Verification items for the finished model (mm, model axes). A direction names the side the tool comes from. Give positions to 0.01 mm unless a question says otherwise; leave off trailing zeros. Loops run counter-clockwise (first coordinate to the right, second up) from the corner with the lowest first, then second, coordinate; pieces in that order, holes last. Notation, with made-up numbers: (78, -22.5) - (87, -22.5) arc R24 cw to (87, -5.5) - close; hole circle Ø9 at (60, -35). An arc over 180 degrees is marked (long way). One line per item, written item: value. Start each with the question number.
1. Mould release check, pull along X, two halves, no side actions. Record for faces 1 (the cylindrical face through (19.961, 48.268, 10.382)), 2 (the flat face through (-3.82, 41.5, -22.34)), 3 (the flat face through (-6, 33, 12)): pulls with the +X half, pulls with the -X half, needs draft (parallel to the pull), parting line crosses it, or undercut.
2. Scan lines: L1, parallel to X at y = 17, z = 0; L2, parallel to X at y = 43, z = 0; L3, parallel to Y at x = 11, z = 22. Record each from-to range of solid material in increasing order. Write a range as [from, to].
3. Sectioned sample at C-C (y = 40.5). Record the cut outline in (x, z).
4. Sectioned sample at A-A (y = 30.5). Record the cut outline in (x, z), plus the area to 3 significant figures.
5. Sectioned sample at B-B (z = 14). Count the separate pieces of the cut face and the enclosed holes in it, plus the area to 3 significant figures.
6. Gauge pin test, flat ends, axial feed: pin 1 (10 mm diameter, centred on x = 16, z = 15.5, fed in from +Y); pin 2 (4 mm diameter, centred on x = 16.5, z = -5.5, fed in from -Y); pin 3 (1.5 mm diameter, centred on x = 12.5, y = 16.5, fed in from -Z). Record the tip position at first contact, or that the pin passes through.
7. Access from +Z, -Z, +X, -X, +Y, -Y to the whole of each face (thin tool, end or side, straight path). Record for faces 4 (the flat face through (-6, 33, -12)), 5 (the cylindrical face through (-0.8, 36.7, 18.4)), 6 (the cylindrical face through (-0.319, 23.257, 17.423)).
from build123d import *

# Parameters (mm, degrees)
CUT_EXTRUDE1_DEPTH       = 70
SKETCH3_R                = 6.25
CUT_EXTRUDE2_DEPTH       = 70
BOSS_EXTRUDE2_REACH      = 78.823
BOSS_EXTRUDE2_END_RADIUS = 23
SKETCH4_R                = 7.25
SKETCH4_R_2              = 6.25


with BuildPart() as part:
    # Sketch1 → Revolve1 (revolve)
    with BuildSketch(Plane.XY, mode=Mode.PRIVATE) as revolve1_sk:
        with BuildLine():
            Line((0, 62.5), (0, 60.49936285))
            ThreePointArc((0, 60.49936285), (12.069492637, 58.859165445), (23, 53.484511145))
            Line((23, 53.484511145), (23, 51.5))
            Line((23, 51.5), (20.5, 51.5))
            Line((20.5, 51.5), (20.5, 45.5))
            Line((20.5, 45.5), (20.5, 39.5))
            Line((20.5, 39.5), (23, 39.5))
            Line((23, 39.5), (23, 0))
            Line((23, 0), (25, 0))
            Line((25, 0), (25, 41.5))
            Line((25, 41.5), (22.5, 41.5))
            Line((22.5, 41.5), (22.5, 44))
            Line((22.5, 44), (25, 44))
            Line((25, 44), (25, 47))
            Line((25, 47), (22.5, 47))
            Line((22.5, 47), (22.5, 49.5))
            Line((22.5, 49.5), (25, 49.5))
            Line((25, 49.5), (25, 54.5))
            ThreePointArc((25, 54.5), (13.174901691, 60.609067785), (0, 62.5))
        make_face()
    revolve(revolve1_sk.sketch.rotate(Axis((0, 62.5, 0), (0, -1, 0)), 90), axis=Axis((0, 62.5, 0), (0, -1, 0)))

    # Sketch2 → Cut-Extrude1 (cut, symmetric)
    with BuildSketch(Plane.XY):
        with BuildLine():
            Line((-19, 0), (19, 0))
            ThreePointArc((19, 0), (0, 9.949493307), (-19, 0))
        make_face()
    extrude(amount=CUT_EXTRUDE1_DEPTH, both=True, mode=Mode.SUBTRACT)

    # Sketch3 → Cut-Extrude2 (cut, symmetric)
    with BuildSketch(Plane.XY):
        with Locations((0, 30.5)):
            Circle(SKETCH3_R)
    extrude(amount=CUT_EXTRUDE2_DEPTH, both=True, mode=Mode.SUBTRACT)

    # Boss-Extrude2: up to this cylinder (the profile starts inside it)
    boss_extrude2_end = Plane(origin=(0, 23.455061, 0), z_dir=(0, 1, 0)) * Cylinder(BOSS_EXTRUDE2_END_RADIUS, 204.646, mode=Mode.PRIVATE)
    # Sketch4 → Boss-Extrude2 (add, up to the surface)
    with BuildSketch(Plane.XY.offset(12), mode=Mode.PRIVATE) as boss_extrude2_sk1:
        with Locations(Location((0, 30.5, 0), (0, 0, 90))):
            Circle(SKETCH4_R)
        with Locations((0, 30.5)):
            Circle(SKETCH4_R_2, mode=Mode.SUBTRACT)
    boss_extrude2_tool1 = extrude(boss_extrude2_sk1.sketch, amount=BOSS_EXTRUDE2_REACH, mode=Mode.PRIVATE) & boss_extrude2_end
    boss_extrude2 = boss_extrude2_tool1.solids().sort_by_distance((0, 23.455061, 12))[0]
    add(boss_extrude2)

    # Mirror1: Boss-Extrude2 across plane
    add(boss_extrude2.mirror(Plane.XY))


solid = part.part
Results are:
1. face 1: parting line crosses it
1. face 2: needs draft
1. face 3: undercut
2. L1: x = [-25, -23], [23, 25]
2. L2: x = [-22.5, -20.5], [20.5, 22.5]
2. L3: y = [7.16, 41.5], [44, 47], [49.5, 54.8]
3. outline: circle Ø50 at (0, 0); hole circle Ø41 at (0, 0)
4. outline: (-7.25, -21.83) arc R23 cw to (-7.25, 21.83) - (-7.25, 12) - (-6.25, 12) - (-6.25, 24.21) arc R25 ccw to (-6.25, -24.21) - (-6.25, -12) - (-7.25, -12) - close; (6.25, -24.21) arc R25 ccw to (6.25, 24.21) - (6.25, 12) - (7.25, 12) - (7.25, 21.83) arc R23 cw to (7.25, -21.83) - (7.25, -12) - (6.25, -12) - close
4. area: 291 mm^2
5. separate pieces: 2
5. enclosed holes: 1
5. area: 442 mm^2
6. pin 1: stops at y = 59.04
6. pin 2: stops at y = 55.76
6. pin 3: stops at z = -22.07
7. face 4: -Y
7. face 5: +Z, -Z
7. face 6: none
